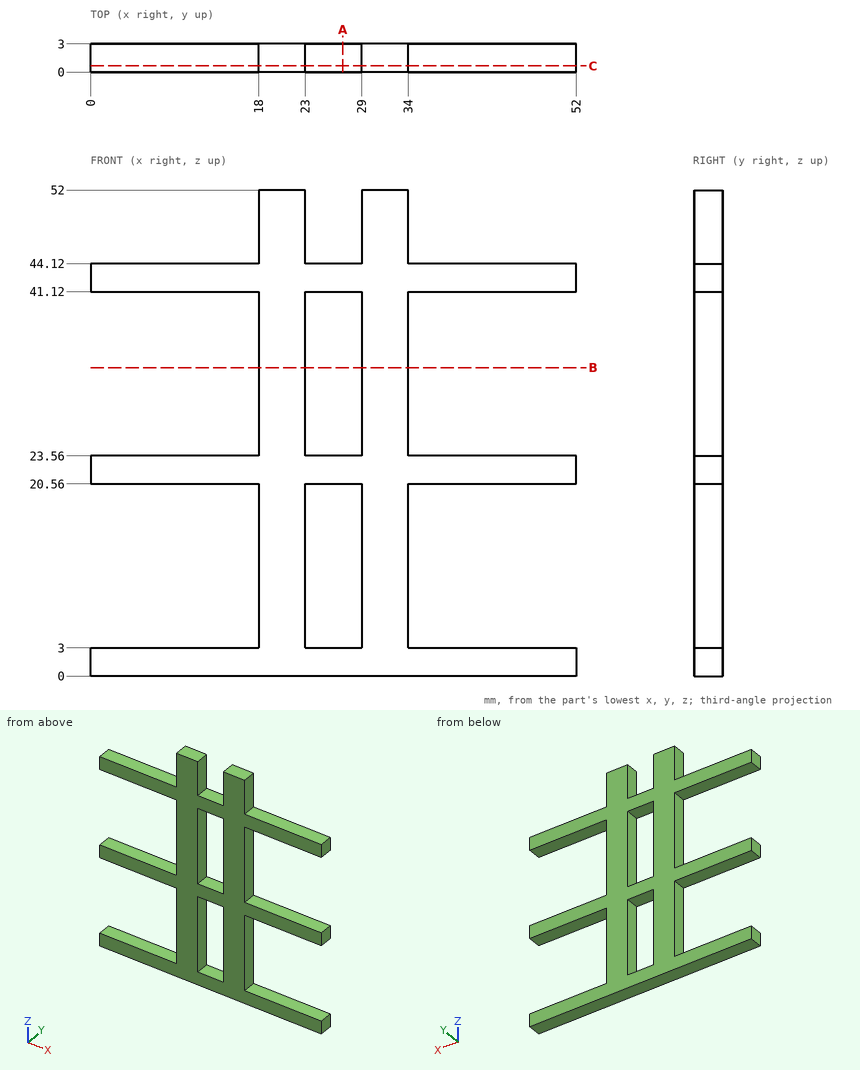
The drawing under review shows one solid part. Ordinate dimensions are in mm from its lowest x, y, z. Give positions to 0.01 mm unless a question says otherwise; leave off trailing zeros. Order: outer loops, then holes, each group sorted by start corner. A loop starts at its lowest first (then second) coordinate and runs counter-clockwise, first axis right, second up. Notation, with made-up numbers: (-4.5, -24) - (38.5, -24) arc R36 cw to (38.5, 13) - close; hole circle Ø10 at (13, 87). An arc over 180 degrees is marked (long way). Answer as a JSON object with one key per item and string values. Group by question number.
Item 1: Take a section at C-C on y = 0.65. Give the number of separate pieces and of enclosed holes in the cut face, and give its area (3 significant figures).
Item 2: Take a section at B-B on z = 33. Give the boundary of the cut face in (x, y), and give its area (3 significant figures).
Item 3: Take a section at A-A on x = 27. Give the boundary of the cut face in (y, z).
Item 4: Clearance check with a flat-ended pin moving along its axis: pin 1 Ø0.9 at (x, y) = (39.5, 1) entering from +Z. State where the tip first meets the part, or that it passes through.
Item 5: Wall thickness on line 1 along Z through (x, y) = (11, 1.6); line 2 along X through (y, z) = (2.6, 47): over which ranges is each line inside the solid? List them lowest first.
Reported:
{
 "1": {"separate pieces": "1", "enclosed holes": "2", "area": "898 mm^2"},
 "2": {"outline": "(18, 0) - (23, 0) - (23, 3) - (18, 3) - close; (29, 0) - (34, 0) - (34, 3) - (29, 3) - close", "area": "30.0 mm^2"},
 "3": {"outline": "(0, 0) - (3, 0) - (3, 3) - (0, 3) - close; (0, 20.56) - (3, 20.56) - (3, 23.56) - (0, 23.56) - close; (0, 41.12) - (3, 41.12) - (3, 44.12) - (0, 44.12) - close"},
 "4": {"pin 1": "z = 44.12"},
 "5": {"line 1": "0 to 3, 20.56 to 23.56, 41.12 to 44.12", "line 2": "18 to 23, 29 to 34"}
}
